Verification items for the finished model (mm, model axes). Face numbers are marked on the shaded views. A direction names the side the tool comes from. Coordinates: 2 decimals unless noted, no trailing zeros. Loops run counter-clockwise (first coordinate to the right, second up) from the corner with the lowest first, then second, coordinate; pieces in that order, holes last.
Q1. Access from +Z, -Z, +X, -X, +Y, -Y to the whole of each face (thin tool, end or side, straight path). Record for the marked faces 1 and 2.
Q2. Sectioned sample at C-C (x = -21). Enter the section's corners in (y, z) (3 decimals).
Q3. Go/stop test with flat-tipped pins: P1, Ø7, axis at y = 12.5, z = 15, coming from the +X side; P2, Ø3, axis at x = -17.5, y = 0, coming from the +Z side (3 decimals); P3, Ø1, axis at y = 11.5, z = 15.5, coming from the +X side. Record where each tip stops, or that it passes through.
Q4. Sectioned sample at A-A (x = 0.5). Enter the section's corners in (y, z), then the cut area to 3 significant figures.
Q5. Material ranges on probe 1 along Y at (x, z) = (1, 19.5); probe 2 along X at (y, z) = (6, 4.5); probe 3 along X at (y, z) = (8.5, 17), recorded low to high.
Q6. Sectioned sample at D-D (y = 11.5). Enter the section's corners in (x, z), then the cut area to 3 significant figures.
Q7. Mould release check, pull along Y, two halves, no side actions. Record for the marked faces 3, 4 and 5: +Y half, -Y half, draft (parallel to the pull), parting line (faces both ways), or undercut.
Q8. Sectioned sample at B-B (z = 12.7). Enter the section's corners in (x, y), then the cut area to 3 significant figures.
```python
from build123d import *

# Parameters (mm, degrees)
F1_DEPTH = 25.4
F2_R     = 6.985
F2_R_2   = 3.81
F3_DEPTH = 2.54
F4_DEPTH = 7


with BuildPart() as f1:
    # F0 (on Top) → F1 (new body)
    with BuildSketch(Plane.XY):
        Polygon((-19.32979, -1.823446), (-19.32979, 21.176554), (6.07021, 21.176554), (6.07021, 25.176554), (-26.32979, 25.176554), (-26.32979, -5.823446), (6.07021, -5.823446), (6.07021, -1.823446), align=None)
    extrude(amount=F1_DEPTH)

    # F2 (on face) → F3 (cut)
    with BuildSketch(Plane.YZ.offset(-19.32979)):
        with Locations((9.676554, 12.7)):
            Circle(F2_R)
        with Locations((9.676554, 12.7)):
            Circle(F2_R_2, mode=Mode.SUBTRACT)
        with Locations((9.676554, 12.7)):
            Circle(F2_R_2)
    extrude(amount=-F3_DEPTH, mode=Mode.SUBTRACT)

    # F2 (on face) → F4 (cut, through all)
    with BuildSketch(Plane.YZ.offset(-19.32979)):
        with Locations((9.676554, 12.7)):
            Circle(F2_R_2)
    extrude(amount=-F4_DEPTH, mode=Mode.SUBTRACT)


solid = f1.part
```
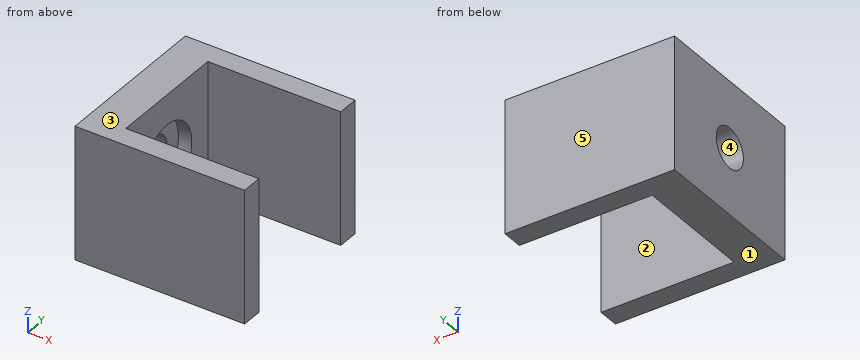
Geometry check:
1. face 1: -Z, +X, -X, +Y, -Y
1. face 2: +Z, -Z, +X
2. outline: (-5.823, 0) - (25.177, 0) - (25.177, 25.4) - (-5.823, 25.4) - close; hole circle Ø13.97 at (9.677, 12.7)
3. P1: stops at x = -19.33
3. P2: passes through
3. P3: stops at x = -21.87
4. outline: (-5.82, 0) - (-1.82, 0) - (-1.82, 25.4) - (-5.82, 25.4) - close; (21.18, 0) - (25.18, 0) - (25.18, 25.4) - (21.18, 25.4) - close
4. area: 203 mm2
5. probe 1: y = -5.82 to -1.82, 21.18 to 25.18
5. probe 2: x = -26.33 to -19.33
5. probe 3: x = -26.33 to -21.87
6. outline: (-26.33, 0) - (-19.33, 0) - (-19.33, 5.96) - (-21.87, 5.96) - (-21.87, 9.35) - (-26.33, 9.35) - close; (-26.33, 16.05) - (-21.87, 16.05) - (-21.87, 19.44) - (-19.33, 19.44) - (-19.33, 25.4) - (-26.33, 25.4) - close
6. area: 114 mm2
7. face 3: draft
7. face 4: undercut
7. face 5: +Y half
8. outline: (-26.33, -5.82) - (6.07, -5.82) - (6.07, -1.82) - (-19.33, -1.82) - (-19.33, 2.69) - (-21.87, 2.69) - (-21.87, 5.87) - (-26.33, 5.87) - close; (-26.33, 13.49) - (-21.87, 13.49) - (-21.87, 16.66) - (-19.33, 16.66) - (-19.33, 21.18) - (6.07, 21.18) - (6.07, 25.18) - (-26.33, 25.18) - close
8. area: 351 mm2
